Here's how the part is built. I have some questions about the finished solid (model axes, mm). A direction names the side the tool comes from. Coordinates: 2 decimals unless noted, no trailing zeros. Write each loop counter-clockwise with the first axis right and the second up, starting at its lowest first coordinate (ties: lowest second). Pieces come first, ordered by that corner, then holes. Notation, with made-up numbers: M -21,86 L 1,86 A29 cw 1,122 Z; hole C -22.5,43 d10. An arc over 180 degrees is marked long. Use one line per item in the form item = value. Start each with the question number.
1. I'm going to push flat-ended pins straight in: pin 1 Ø0.8 at (x, z) = (-13.5, 15.5) entering from -Y; pin 2 Ø3 at (x, y) = (-17, -1) entering from -Z; pin 3 Ø2 at (x, z) = (-16.5, 11.5) entering from -Y; pin 4 Ø10 at (x, z) = (-8.5, 17) entering from -Y. Where does each tip first touch, or does it pass through?
2. I want a section at B-B, the plane x = 3.75. List the corners of the cut face in (y, z) for me.
3. Thinking about a two-plate mould opening in X: for faces 4 (the face through (5.266, 6, 13)), 5 (the face through (-1.155, 5.073, 13.311)), 6 (the face through (-18.734, -2, 4)), which applies, released by +X, released by -X, zero draft, split by the parting line, or undercut?
4. Please list where these lines run through material, in increasing order: line 1 along Z through (x, y) = (-17, -4); line 2 along Y through (x, z) = (-3.5, 5.75); line 3 along Y through (x, z) = (-2.25, 16). Write a range as [from, to].
5. I want a section at D-D, the plane z = 6. List the corners of the cut face in (x, y) for me.
6. I want a section at C-C, the plane y = -3.5. List the corners of the cut face in (x, z) for me.
7. On a 3-axis mill with a long thin cutter (end or side, diameter ignored), from which of +Z, -Z, +X, -X, +Y, -Y can I reach the whole of each face in a straight line? I mean faces 1 (the face through (-12.734, 0, 9)), 2 (the face through (-13, -1, 23)), 3 (the face through (-15, 1, 23)). Say none if no direction works.
8. I want a section at A-A, the plane x = -16. List the corners of the cut face in (y, z) for me.
from build123d import *

# Parameters (mm, degrees)
BOSS_EXTRU_1_DEPTH      = 27
ESQUISSE2_W             = 1.5
ESQUISSE2_H             = 20
ENL_V_MAT_EXTRU_3_DEPTH = 6
CONG_1_R                = 1


with BuildPart() as part:
    # Esquisse1 → Boss.-Extru.1 (new body)
    with BuildSketch(Plane.XY):
        with BuildLine():
            Line((-12.734069529, 1), (-18.734069529, 1))
            Line((-18.734069529, 1), (-18.734069529, -5))
            Line((-18.734069529, -5), (-14.734069529, -5))
            Line((-14.734069529, -5), (-14.734069529, -1))
            Line((-14.734069529, -1), (-12.734069529, -1))
            ThreePointArc((-12.734069529, -1), (-4.80129438, -7.212987875), (5.265930471, -7.638574159))
            Line((5.265930471, -7.638574159), (5.265930471, -4.5))
            ThreePointArc((5.265930471, -4.5), (-1.066525943, -5.086207973), (-6.961264916, -2.69964214))
            ThreePointArc((-6.961264916, -2.69964214), (-8.345527914, 0), (-6.961264916, 2.69964214))
            ThreePointArc((-6.961264916, 2.69964214), (-1.066525943, 5.086207973), (5.265930471, 4.5))
            Line((5.265930471, 4.5), (5.265930471, 7.638574159))
            ThreePointArc((5.265930471, 7.638574159), (-4.80129438, 7.212987875), (-12.734069529, 1))
        make_face()
    extrude(amount=BOSS_EXTRU_1_DEPTH)

    # Esquisse2 → Enlèv. mat.-Extru.3 (cut)
    with BuildSketch(Plane.ZY.offset(18.734069529)):
        with Locations((8.75, 1.023656904)):
            Rectangle(ESQUISSE2_W, ESQUISSE2_H)
        with Locations((18.25, 1)):
            Rectangle(ESQUISSE2_W, ESQUISSE2_H)
    extrude(amount=-ENL_V_MAT_EXTRU_3_DEPTH, mode=Mode.SUBTRACT)

    # Congé1
    cong_1_edges = [part.edges().sort_by_distance(p)[0] for p in [
        (-14.734069529, -1, 23),
        (-18.734069529, 1, 23),
        (-14.734069529, -1, 13.5),
        (-14.734069529, -1, 4),
        (-18.734069529, 1, 13.5),
        (-18.734069529, 1, 4),
    ]]
    fillet(cong_1_edges, radius=CONG_1_R)


solid = part.part
Answer list:
q1.pin_1 = -1.01
q1.pin_2 = 0
q1.pin_3 = -5
q1.pin_4 = -7.63
q2.outline = M -7.98,0 L -4.92,0 L -4.92,27 L -7.98,27 Z; M 4.92,0 L 7.98,0 L 7.98,27 L 4.92,27 Z
q3.face_4 = released by +X
q3.face_5 = undercut
q3.face_6 = released by -X
q4.line_1 = [0, 8], [9.5, 17.5], [19, 27]
q4.line_2 = [-7.63, -4.49], [4.49, 7.63]
q4.line_3 = [-7.93, -4.86], [4.86, 7.93]
q5.outline = M -18.73,-5 L -14.73,-5 L -14.73,-2 A1 cw -13.73,-1 L -12.73,-1 A16.46 ccw 5.27,-7.64 L 5.27,-4.5 A13.46 cw -6.96,-2.7 A3.32 cw -6.96,2.7 A13.46 cw 5.27,4.5 L 5.27,7.64 A16.46 ccw -12.73,1 L -17.73,1 A1 ccw -18.73,0 Z
q6.outline = M -18.73,0 L -14.73,0 L -14.73,8 L -18.73,8 Z; M -18.73,9.5 L -14.73,9.5 L -14.73,17.5 L -18.73,17.5 Z; M -18.73,19 L -14.73,19 L -14.73,27 L -18.73,27 Z; M -10.65,0 L -5.71,0 L -5.71,27 L -10.65,27 Z
q7.face_1 = -X, +Y, -Y
q7.face_2 = +Z, -Z, -Y
q7.face_3 = +Z, -Z, -X, +Y
q8.outline = M -5,0 L 1,0 L 1,8 L -5,8 Z; M -5,9.5 L 1,9.5 L 1,17.5 L -5,17.5 Z; M -5,19 L 1,19 L 1,27 L -5,27 Z
